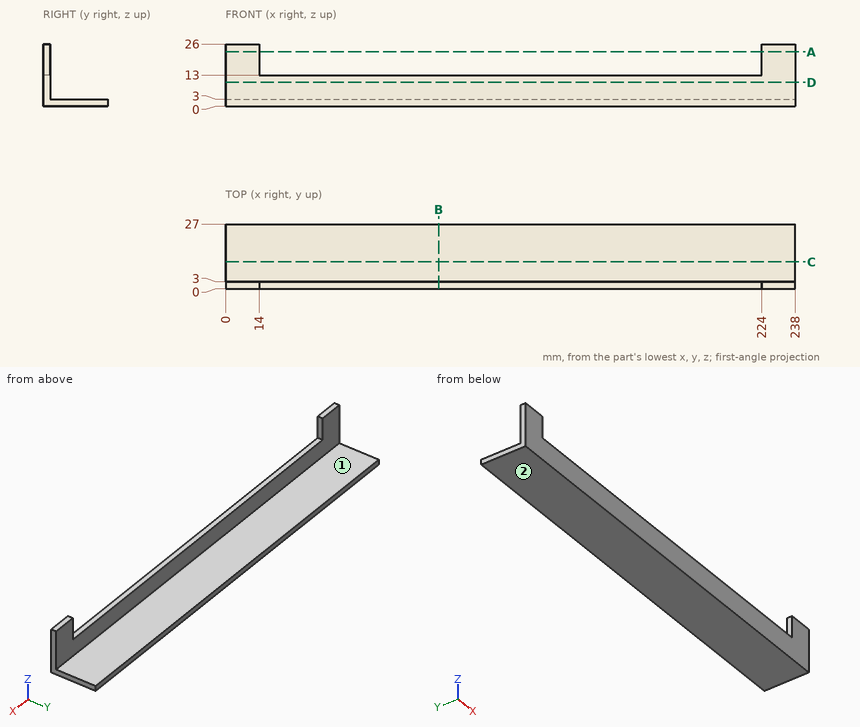
For this review, use the dimensioned drawing (mm, ordinates from the lowest corner) and the shaded views. A direction names the side the tool comes from. Give positions to 0.01 mm unless a question says otherwise; leave off trailing zeros. Order: outer loops, then holes, each group sorted by start corner. A loop starts at its lowest first (then second) coordinate and runs counter-clockwise, first axis right, second up. Notation, with made-up numbers: M -3.75,83 L 45.25,83 A12 ccw 45.25,93 Z; hole C 33.25,79 d8. An arc over 180 degrees is marked long. Use one line per item in the form item = value. Start each with the question number.
Item 1: We need section C-C on y = 11.25. Give the boundary of the cut face in (x, z), plus the area to 3 significant figures.
Item 2: We need section B-B on x = 89. Give the boundary of the cut face in (y, z), plus the area to 3 significant figures.
Item 3: To check wall thickness, follow line 1 along Z through (x, y) = (28, 22); line 2 along Z through (x, y) = (44.5, 1.25). State the ranges of each line that lie inside material, in increasing order. Write a range as from..to.
Item 4: For the marked faces 1 and 2, list the 3-axis set-ups (+Z, -Z, +X, -X, +Y, -Y) from which the entire face can be reached by the end or side of a thin tool; tool diameter is ignored.
Item 5: We need section A-A on z = 22.75. Give the boundary of the cut face in (x, y), plus the area to 3 significant figures.
Item 6: Insertion check: pin 1 Ø6 at (x, z) = (142.5, 4) entering from -Y; pin 2 Ø0.9 at (x, y) = (146, 2) entering from +Z; pin 3 Ø4 at (x, y) = (52.5, 21) entering from +Z. Each pin has a flat end and moves straight along its axis. Give the tip position at first contact, or say it passes through.
Completed:
q1.outline = M 0,0 L 238,0 L 238,3 L 0,3 Z
q1.area = 714 mm²
q2.outline = M 0,0 L 27,0 L 27,3 L 3,3 L 3,13 L 0,13 Z
q2.area = 111 mm²
q3.line_1 = 0..3
q3.line_2 = 0..13
q4.face_1 = +Z, +X, -X, +Y
q4.face_2 = -Z, +X, -X, +Y, -Y
q5.outline = M 0,0 L 14,0 L 14,3 L 0,3 Z; M 224,0 L 238,0 L 238,3 L 224,3 Z
q5.area = 84.0 mm²
q6.pin_1 = 0
q6.pin_2 = 13
q6.pin_3 = 3
